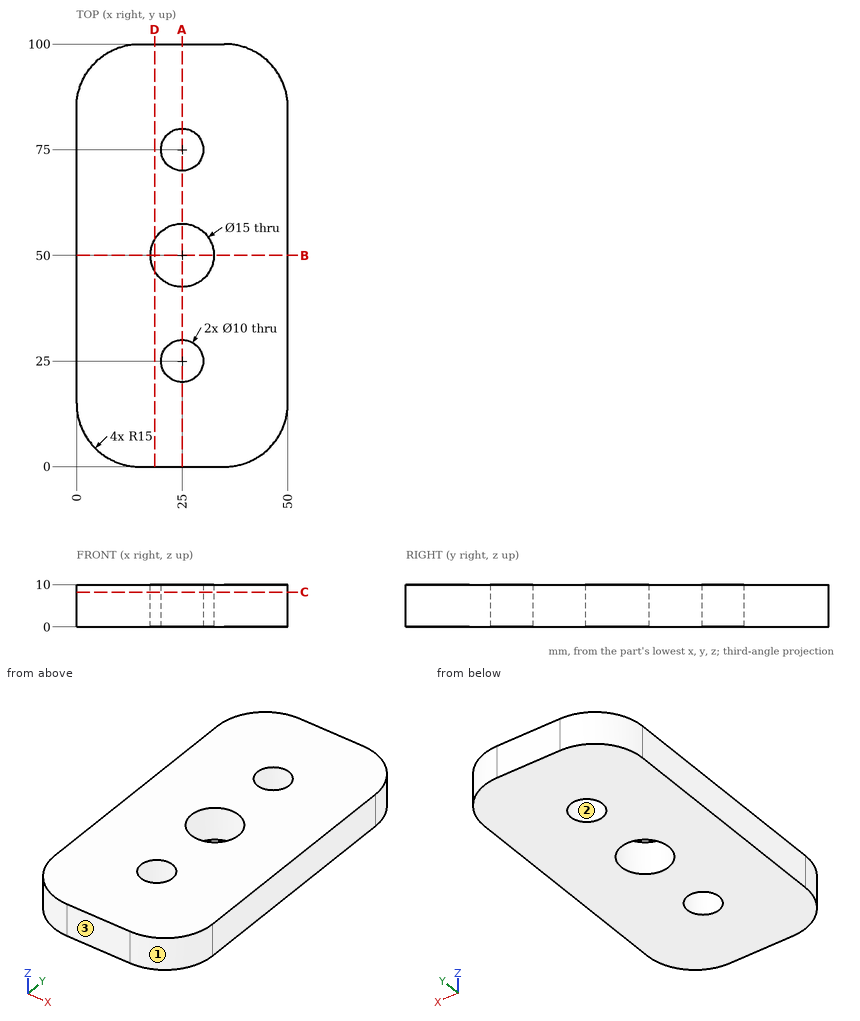
Geometry: see drawing. Coordinates: mm, zero at the bounding-box minimum. Coordinates: 2 decimals unless noted, no trailing zeros. Order: outer loops, then holes, each group sorted by start corner. A loop starts at its lowest first (then second) coordinate and runs counter-clockwise, first axis right, second up. Notation, with made-up numbers: (-32, 23.5) - (0, 23.5) arc R17 ccw to (0, 50.5) - close; hole circle Ø4 at (6, -2.75). An arc over 180 degrees is marked (long way). Return JSON: item names as keys, results as strings.
Q1. Draft query along X for the marked faces 1, 2 and 3. Return one class per face: +X half, -X half, draft (parallel to the pull), parting line (faces both ways), or undercut.
The answers:
{"face 1": "+X half", "face 2": "undercut", "face 3": "draft"}
Q2. Cut plane C-C (z = 8.25). Return loops of the section in (x, y).
The answers:
{"outline": "(0, 15) arc R15 ccw to (15, 0) - (35, 0) arc R15 ccw to (50, 15) - (50, 85) arc R15 ccw to (35, 100) - (15, 100) arc R15 ccw to (0, 85) - close; hole circle Ø15 at (25, 50); hole circle Ø10 at (25, 25); hole circle Ø10 at (25, 75)"}
Q3. Cut plane A-A (x = 25). Return loops of the section in (y, z).
The answers:
{"outline": "(0, 0) - (20, 0) - (20, 10) - (0, 10) - close; (30, 0) - (42.5, 0) - (42.5, 10) - (30, 10) - close; (57.5, 0) - (70, 0) - (70, 10) - (57.5, 10) - close; (80, 0) - (100, 0) - (100, 10) - (80, 10) - close"}
Q4. First-contact query: pin 1 (1.5 mm diameter, centred on x = 36.5, z = 3, fed in from +Y); pin 2 (5 mm diameter, centred on x = 8.5, z = 2.5, fed in from -Y). Flat tips, straight axial feed; report the tip coordinate or a pass-through.
The answers:
{"pin 1": "stops at y = 99.98", "pin 2": "stops at y = 0.54"}
Q5. Cut plane D-D (x = 18.5). Return loops of the section in (y, z), then the cut area to 3 significant figures.
The answers:
{"outline": "(0, 0) - (46.26, 0) - (46.26, 10) - (0, 10) - close; (53.74, 0) - (100, 0) - (100, 10) - (53.74, 10) - close", "area": "925 mm2"}
Q6. Ray query, probe 1 along Y at (x, z) = (25, 3.25); probe 2 along Y at (x, z) = (26, 4.75); probe 3 along X at (y, z) = (49, 4.5). Return the intervals inside material, ascending.
The answers:
{"probe 1": "y = 0 to 20, 30 to 42.5, 57.5 to 70, 80 to 100", "probe 2": "y = 0 to 20.1, 29.9 to 42.57, 57.43 to 70.1, 79.9 to 100", "probe 3": "x = 0 to 17.57, 32.43 to 50"}
Q7. Cut plane B-B (y = 50). Return loops of the section in (x, z).
The answers:
{"outline": "(0, 0) - (17.5, 0) - (17.5, 10) - (0, 10) - close; (32.5, 0) - (50, 0) - (50, 10) - (32.5, 10) - close"}
